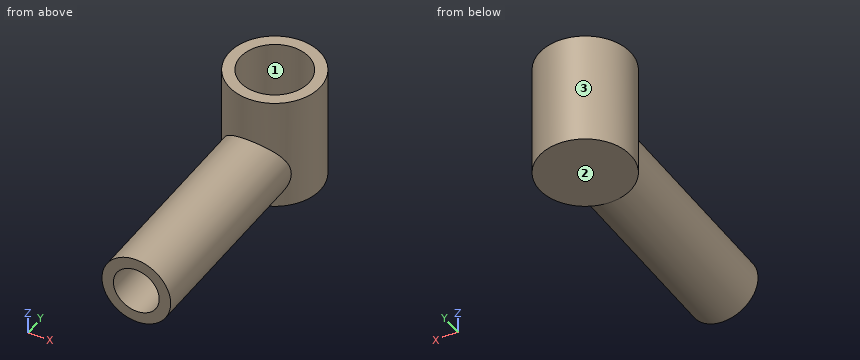
```python
from build123d import *

# Parameters (mm, degrees)
ESQUISSE1_R             = 4
BOSS_EXTRU_1_DEPTH      = 8
BOSS_EXTRU_1_DEPTH_BACK = 2
ESQUISSE4_R             = 2
ENL_V_MAT_EXTRU_2_DEPTH = 18
BOSS_EXTRU_2_START      = -2.5
ESQUISSE3_R             = 3
ESQUISSE3_R_2           = 2
BOSS_EXTRU_2_DEPTH      = 1
BOSS_EXTRU_2_DEPTH_BACK = 18
ESQUISSE2_R             = 3
ENL_V_MAT_EXTRU_3_DEPTH = 9


with BuildPart() as part:
    # Esquisse1 → Boss.-Extru.1 (new body, two sides)
    with BuildSketch(Plane.XY) as boss_extru_1_sk:
        Circle(ESQUISSE1_R)
    extrude(amount=BOSS_EXTRU_1_DEPTH)
    extrude(boss_extru_1_sk.sketch, amount=-BOSS_EXTRU_1_DEPTH_BACK)

    # Esquisse4 → Enlèv. mat.-Extru.2 (cut)
    with BuildSketch(Plane(origin=(0, 0, 0), x_dir=(1, 0, 0), z_dir=(0, 1, 0))):
        with Locations((0, -1)):
            Circle(ESQUISSE4_R)
    extrude(amount=-ENL_V_MAT_EXTRU_2_DEPTH, mode=Mode.SUBTRACT)

    # Esquisse3 → Boss.-Extru.2 (add, two sides)
    with BuildSketch(Plane(origin=(0, 0, 0), x_dir=(1, 0, 0), z_dir=(0, 1, 0)).offset(BOSS_EXTRU_2_START)) as boss_extru_2_sk:
        with Locations((0, -1)):
            Circle(ESQUISSE3_R)
        with Locations((0, -1)):
            Circle(ESQUISSE3_R_2, mode=Mode.SUBTRACT)
    extrude(amount=BOSS_EXTRU_2_DEPTH)
    extrude(boss_extru_2_sk.sketch, amount=-BOSS_EXTRU_2_DEPTH_BACK)

    # Esquisse2 → Enlèv. mat.-Extru.3 (cut)
    with BuildSketch(Plane.XY.offset(8)):
        Circle(ESQUISSE2_R)
    extrude(amount=-ENL_V_MAT_EXTRU_3_DEPTH, mode=Mode.SUBTRACT)


solid = part.part
```
CAD build for the part. Positions are in the model's coordinates, mm. Face numbers are marked on the shaded views. Round coordinates to 2 decimals unless told otherwise and drop trailing zeros. Order: outer loops, then holes, each group sorted by start corner. A loop starts at its lowest first (then second) coordinate and runs counter-clockwise, first axis right, second up. Notation, with made-up numbers: (36.5, -25) - (51.5, -25) arc R8 cw to (51.5, -13) - close; hole circle Ø8 at (-11.75, 31.5). An arc over 180 degrees is marked (long way). Answer in a Markdown table with one row per item. Add a question column.
(1) Band-saw the part on A-A on x = 0.75. List the corners of the cut face in (y, z).
(2) Probe L1, parallel to X at y = -10.75, z = 1; L2, parallel to X at y = 0, z = 2.5; L3, parallel to Z at x = 0, y = -3.3. List the from-to ranges inside material, lowest first. Write a range as [from, to].
(3) Band-saw the part on D-D on y = 0. List the corners of the cut face in (x, z).
(4) Band-saw the part on C-C on y = -16.25. List the corners of the cut face in (x, z), and give its area (3 significant figures).
(5) Drop flat-ended pins along their axis: pin 1 Ø3.5 at (x, y) = (0, 0) entering from +Z; pin 2 Ø2 at (x, y) = (1.5, -17) entering from -Z; pin 3 Ø2.5 at (x, z) = (0, 1) entering from -Y; pin 4 Ø3 at (x, z) = (-3, -0.5) entering from -Y. Give the stop position or say it passes through.
(6) Mould opens along Y. For the marked faces 1, 2 and 3 say: +Y half, -Y half, draft (parallel to the pull), parting line (faces both ways), or undercut.
(7) Band-saw the part on B-B on z = 1. List the corners of the cut face in (x, y).
Data:
| question | item | result |
|---|---|---|
| 1 | outline | (-20.5, -1.9) - (-3.93, -1.9) - (-3.93, -2) - (3.93, -2) - (3.93, 8) - (2.9, 8) - (2.9, -1) - (-2.9, -1) - (-2.9, -0.85) - (-20.5, -0.85) - close; (-20.5, 2.85) - (-2.9, 2.85) - (-2.9, 8) - (-3.93, 8) - (-3.93, 3.9) - (-20.5, 3.9) - close |
| 2 | L1 | x = [-3, -2], [2, 3] |
| 2 | L2 | x = [-4, -3], [3, 4] |
| 2 | L3 | z = [-2, -1], [3, 8] |
| 3 | outline | (-4, -2) - (4, -2) - (4, 8) - (3, 8) - (3, -1) - (-3, -1) - (-3, 8) - (-4, 8) - close |
| 4 | outline | circle Ø6 at (0, 1); hole circle Ø4 at (0, 1) |
| 4 | area | 15.7 mm^2 |
| 5 | pin 1 | stops at z = -1 |
| 5 | pin 2 | stops at z = -1.96 |
| 5 | pin 3 | stops at y = 2.73 |
| 5 | pin 4 | stops at y = -20.5 |
| 6 | face 1 | undercut |
| 6 | face 2 | draft |
| 6 | face 3 | parting line |
| 7 | outline | (-3, -20.5) - (-2, -20.5) - (-2, -2.24) arc R3 cw (long way) to (2, -2.24) - (2, -20.5) - (3, -20.5) - (3, -2.65) arc R4 ccw (long way) to (-3, -2.65) - close |
